Input: part model. Units: mm. Frame: model coordinates. Give positions to 0.01 mm unless a question says otherwise; leave off trailing zeros. Loops run counter-clockwise (first coordinate to the right, second up) from the corner with the lowest first, then second, coordinate; pieces in that order, holes last. Notation, with made-up numbers: (88.25, -1) -> (144.25, -1) arc R20 cw to (144.25, 19) -> close; hole circle Ø10 at (83, 33). An arc over 180 degrees is marked (long way). Answer as a JSON object with one key per item and string values.
```python
from build123d import *

# Parameters (mm, degrees)
CYLINDER_R          = 5
CYLINDER_DEPTH      = 20
CYLINDER_ROLL_ANGLE = 90
BOX_W               = 24
BOX_H               = 14
BOX_DEPTH           = 5
SKETCH001_R         = 1.95
POCKET_DEPTH        = 15
FILLET_R            = 2
CHAMFER_SIZE        = 0.2
CHAMFER001_SIZE     = 0.2


with BuildPart() as zylinder:
    # Cylinder → Cylinder (new body)
    with BuildSketch(Plane.XY):
        Circle(CYLINDER_R)
    extrude(amount=CYLINDER_DEPTH)


with BuildPart() as zylinder_1:
    # Cylinder roll: moved
    add(zylinder.part.rotate(Axis((0, 0, 0), (1, 0, 0)), CYLINDER_ROLL_ANGLE))


with BuildPart() as zylinder_2:
    # Cylinder placement: moved
    add(zylinder_1.part.moved(Location((0, 10, -2))))


with BuildPart() as chamfer001:
    # Box → Box (new body)
    with BuildSketch(Plane(origin=(-12, -7, 0), x_dir=(1, 0, 0), z_dir=(0, 0, 1))):
        with Locations((12, 7)):
            Rectangle(BOX_W, BOX_H)
    extrude(amount=BOX_DEPTH)

    # Cut: cut Zylinder
    add(zylinder_2.part, mode=Mode.SUBTRACT)

    # Sketch001 → Pocket (cut)
    with BuildSketch(Plane(origin=(0, 0, 0), x_dir=(1, 0, 0), z_dir=(0, 0, -1))):
        with Locations((-7.5, 0)):
            Circle(SKETCH001_R)
        with Locations((7.5, 0)):
            Circle(SKETCH001_R)
    extrude(amount=-POCKET_DEPTH, mode=Mode.SUBTRACT)

    # Fillet
    fillet_edges = [chamfer001.edges().sort_by_distance(p)[0] for p in [
        (-12, 7, 2.5),
        (-12, -7, 2.5),
        (12, -7, 2.5),
        (12, 7, 2.5),
    ]]
    fillet(fillet_edges, radius=FILLET_R)

    # Chamfer
    chamfer_edges = [chamfer001.edges().sort_by_distance(p)[0] for p in [
        (-12, 0, 0),
        (-11.414214, 6.414214, 0),
        (-7.291288, 7, 0),
        (-4.582576, 0, 0),
        (-7.291288, -7, 0),
        (-11.414214, -6.414214, 0),
        (4.582576, 0, 0),
        (7.291288, -7, 0),
        (11.414214, -6.414214, 0),
        (12, 0, 0),
        (11.414214, 6.414214, 0),
        (7.291288, 7, 0),
        (-9.45, 0, 0),
        (5.55, 0, 0),
    ]]
    chamfer(chamfer_edges, length=CHAMFER_SIZE)

    # Chamfer001
    chamfer001_edges = [chamfer001.edges().sort_by_distance(p)[0] for p in [
        (0, 7, 5),
        (11.414214, 6.414214, 5),
        (12, 0, 5),
        (11.414214, -6.414214, 5),
        (0, -7, 5),
        (-11.414214, -6.414214, 5),
        (-12, 0, 5),
        (-11.414214, 6.414214, 5),
        (-9.45, 0, 5),
        (5.55, 0, 5),
    ]]
    chamfer(chamfer001_edges, length=CHAMFER001_SIZE)


solid = chamfer001.part
```
Q1. Section B-B, the plane x = 7.5. Return the cut outline in (y, z), then the cut area to 3 significant figures.
Evaluation:
{"outline": "(-7, 0.2) -> (-6.8, 0) -> (-2.15, 0) -> (-1.95, 0.2) -> (-1.95, 4.8) -> (-2.15, 5) -> (-6.8, 5) -> (-7, 4.8) -> close; (1.95, 0.2) -> (2.15, 0) -> (6.8, 0) -> (7, 0.2) -> (7, 4.8) -> (6.8, 5) -> (2.15, 5) -> (1.95, 4.8) -> close", "area": "50.3 mm2"}
Q2. Section D-D, the plane z = 4.55. Return the cut outline in (x, y).
Evaluation:
{"outline": "(-12, -5) arc R2 ccw to (-10, -7) -> (10, -7) arc R2 ccw to (12, -5) -> (12, 5) arc R2 ccw to (10, 7) -> (-10, 7) arc R2 ccw to (-12, 5) -> close; hole circle Ø3.9 at (-7.5, 0); hole circle Ø3.9 at (7.5, 0)"}
Q3. Ray query, line 1 along X through (y, z) = (0, 3.4); line 2 along X through (y, z) = (0, 2.15); line 3 along X through (y, z) = (-1.5, 0.3). Return the intervals inside material, ascending.
Evaluation:
{"line 1": "x = -12 to -9.45, -5.55 to 5.55, 9.45 to 12", "line 2": "x = -12 to -9.45, -5.55 to -2.79, 2.79 to 5.55, 9.45 to 12", "line 3": "x = -12 to -8.75, -6.25 to -4.44, 4.44 to 6.25, 8.75 to 12"}
Q4. Section A-A, the plane y = 0. Return the cut outline in (x, z), then the cut area to 3 significant figures.
Evaluation:
{"outline": "(-12, 0.2) -> (-11.8, 0) -> (-9.65, 0) -> (-9.45, 0.2) -> (-9.45, 4.8) -> (-9.65, 5) -> (-11.8, 5) -> (-12, 4.8) -> close; (-5.55, 0.2) -> (-5.35, 0) -> (-4.78, 0) -> (-4.5, 0.18) arc R5 cw to (4.5, 0.18) -> (4.78, 0) -> (5.35, 0) -> (5.55, 0.2) -> (5.55, 4.8) -> (5.35, 5) -> (-5.35, 5) -> (-5.55, 4.8) -> close; (9.45, 0.2) -> (9.65, 0) -> (11.8, 0) -> (12, 0.2) -> (12, 4.8) -> (11.8, 5) -> (9.65, 5) -> (9.45, 4.8) -> close", "area": "60.9 mm2"}
Q5. Section C-C, the plane z = 1.3. Return the cut outline in (x, y), then the cut area to 3 significant figures.
Evaluation:
{"outline": "(-12, -5) arc R2 ccw to (-10, -7) -> (-3.76, -7) -> (-3.76, 7) -> (-10, 7) arc R2 ccw to (-12, 5) -> close; (3.76, -7) -> (10, -7) arc R2 ccw to (12, -5) -> (12, 5) arc R2 ccw to (10, 7) -> (3.76, 7) -> close; hole circle Ø3.9 at (-7.5, 0); hole circle Ø3.9 at (7.5, 0)", "area": "203 mm2"}
Q6. Draft query along X for faces 1 (the flat face through (-0.1, -7, 3.5)), 2 (the cylindrical face through (5.552, -0.086, 2.468)), 3 (the cylindrical face through (11.4, -6.43, 2.53)). Return one class per face: +X half, -X half, draft (parallel to the pull), parting line (faces both ways), or undercut.
Evaluation:
{"face 1": "draft", "face 2": "undercut", "face 3": "+X half"}
